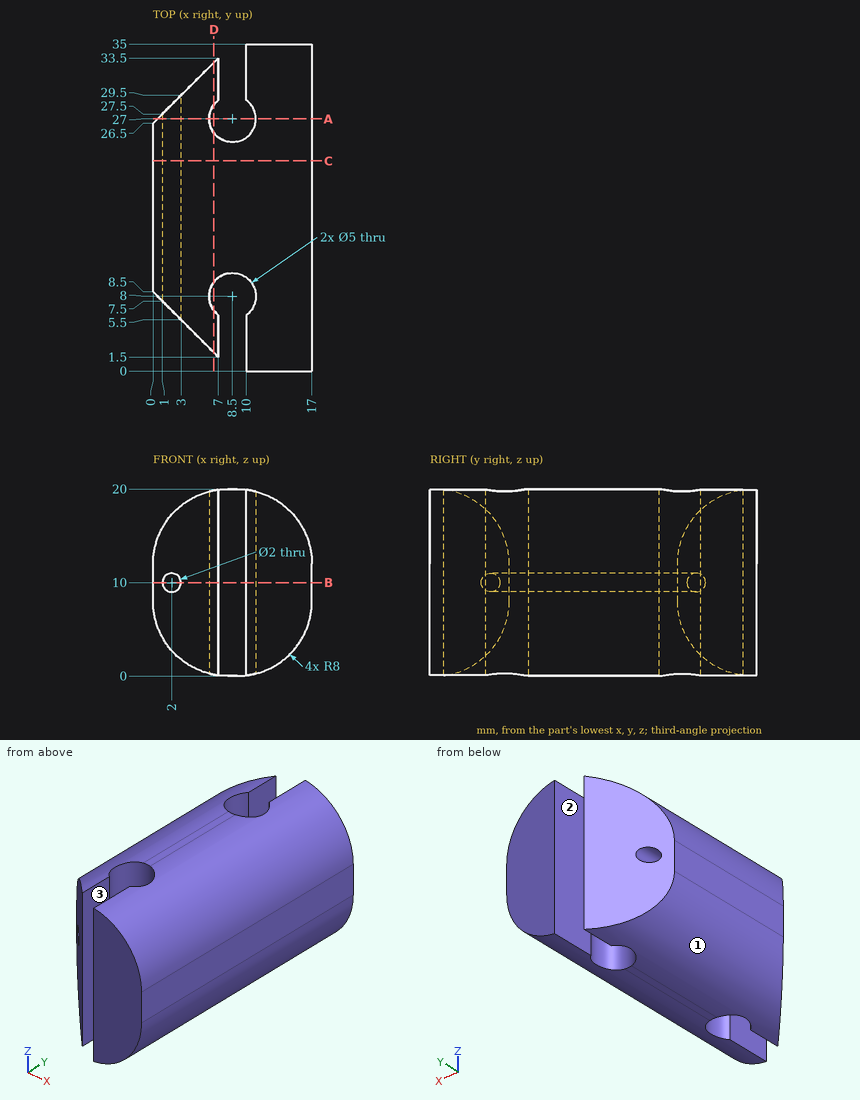
Geometry: see drawing. Coordinates: mm, zero at the bounding-box minimum. A direction names the side the tool comes from. Give positions to 0.01 mm unless a question says otherwise; leave off trailing zeros. Order: outer loops, then holes, each group sorted by start corner. A loop starts at its lowest first (then second) coordinate and runs counter-clockwise, first axis right, second up. Notation, with made-up numbers: M 26.5,5 L 41.5,5 A10 cw 41.5,19 Z; hole C 19,7 d11. An arc over 180 degrees is marked long. Answer as a JSON object with one key per item and string values.
1. Reachability of the marked faces 1, 2 and 3 from +Z, -Z, +X, -X, +Y, -Y: full face, straight path, thin tool, end or side. Return the list, or none.
Result sheet:
{"face 1": "-Z, -X, +Y, -Y", "face 2": "+Z, -Z, +Y", "face 3": "+Z, -Z, -Y"}
2. Ray query, line 1 (X direction, y = 32, z = 10); line 2 (Y direction, x = 10.25, z = 7); line 3 (Z direction, x = 2, y = 18). Return the intervals inside material, ascending. Write a range as [from, to].
Result sheet:
{"line 1": "[5.5, 7], [10, 17]", "line 2": "[0, 6.21], [9.79, 25.21], [28.79, 35]", "line 3": "[2.71, 9], [11, 17.29]"}
3. Cut plane A-A, the plane y = 27. Output: boundary loops of the cut face in (x, z), and give its area (3 significant figures).
Result sheet:
{"outline": "M 0.5,5.22 A8 ccw 6,0.25 L 6,19.75 A8 ccw 0.5,14.78 Z; M 11,0.25 A8 ccw 17,8 L 17,12 A8 ccw 11,19.75 Z; hole C 2,10 d2", "area": "179 mm²"}
4. Cut plane B-B, the plane z = 10. Output: boundary loops of the cut face in (x, y), and give its area (3 significant figures).
Result sheet:
{"outline": "M 0,8.5 L 1,7.5 L 1,27.5 L 0,26.5 Z; M 3,5.5 L 7,1.5 L 7,6 A2.5 cw long 10,6 L 10,0 L 17,0 L 17,35 L 10,35 L 10,29 A2.5 cw long 7,29 L 7,33.5 L 3,29.5 Z", "area": "408 mm²"}
5. Cut plane D-D, the plane x = 6.5. Output: boundary loops of the cut face in (y, z), and give its area (3 significant figures).
Result sheet:
{"outline": "M 2,0.14 L 6.5,0.14 L 6.5,19.86 L 2,19.86 Z; M 9.5,0.14 L 25.5,0.14 L 25.5,19.86 L 9.5,19.86 Z; M 28.5,0.14 L 33,0.14 L 33,19.86 L 28.5,19.86 Z", "area": "493 mm²"}
6. Cut plane C-C, the plane y = 22.5. Output: boundary loops of the cut face in (x, z).
Result sheet:
{"outline": "M 0,8 A8 ccw 8,0 L 9,0 A8 ccw 17,8 L 17,12 A8 ccw 9,20 L 8,20 A8 ccw 0,12 Z; hole C 2,10 d2"}
7. First-contact query: P1, Ø5, axis at y = 30.5, z = 15, coming from the +X side; P2, Ø3, axis at x = 8.5, y = 27, coming from the -Z side; P3, Ø3, axis at x = 13, y = 17, coming from the -Z side; P4, Ø1.5, axis at y = 5.5, z = 5, coming from the -X side. Flat tips, straight axial feed; report the tip coordinate or a pass-through.
Result sheet:
{"P1": "x = 16.98", "P2": "through", "P3": "z = 0.4", "P4": "x = 2.25"}
